For this review, take the finished solid that the model builds, in its own axes (mm). Face numbers are marked on the shaded views. Coordinates: 2 decimals unless noted, no trailing zeros. Answer as a JSON object with one key per item and string values. Group by question number.
Item 1: Clearance check with flat-ended pins moving along their axes: pin 1 (3 mm diameter, centred on x = -120.5, z = 50, fed in from +Y); pin 2 (1 mm diameter, centred on x = 18, z = -11, fed in from -Y). State where each tip first meets the part, or that it passes through.
Item 2: Mouldability with a two-part tool opening along Z and no side actions: class the marked faces 1 and 2 as released by +Z, released by -Z, zero draft, split by the parting line, or undercut.
Item 3: To check wall thickness, follow line 1 (Y direction, x = -121.5, z = 17); line 2 (Z direction, x = -61.5, y = -18); line 3 (X direction, y = -15.5, z = 8). State the ranges of each line that lie inside material, in increasing order.
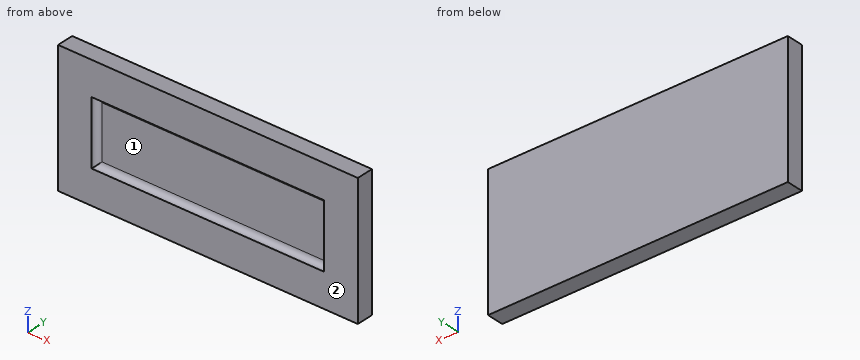
from build123d import *

# Parameters (mm, degrees)
F0_W     = 339.725
F0_H     = 149.225
F0_W_2   = 263.525
F0_H_2   = 73.025
F1_DEPTH = 19.05
F2_DEPTH = 12.7
F3_R     = 6.34999


# Not quite as in the source:
# - a fillet or chamfer is up to 0.001 mm smaller than in the source, because OpenCascade refuses the exact size


with BuildPart() as f1:
    # F0 (on Front) → F1 (new body)
    with BuildSketch(Plane.XZ):
        Rectangle(F0_W, F0_H)
        Rectangle(F0_W_2, F0_H_2, mode=Mode.SUBTRACT)
    extrude(amount=F1_DEPTH)

    # F0 (on Front) → F2 (join)
    with BuildSketch(Plane.XZ):
        Rectangle(F0_W_2, F0_H_2)
    extrude(amount=F2_DEPTH)

    # F3 (radius 6.35 in the source; OpenCascade refuses exactly that, so slightly less here)
    f3_edges = [f1.edges().sort_by_distance(p)[0] for p in [
        (0, -12.7, 36.5125),
        (-131.7625, -12.7, 0),
        (0, -12.7, -36.5125),
        (131.7625, -12.7, 0),
    ]]
    fillet(f3_edges, radius=F3_R)


solid = f1.part
Check sheet entries:
{
 "1": {"pin 1": "stops at y = 0", "pin 2": "stops at y = -12.7"},
 "2": {"face 1": "undercut", "face 2": "zero draft"},
 "3": {"line 1": "y = -12.7 to 0", "line 2": "z = -74.61 to -36.43, 36.43 to 74.61", "line 3": "x = -169.86 to -130.68, 130.68 to 169.86"}
}
